Source: CAD feature listing. Evaluate the final solid. Frame: model axes, mm. A direction names the side the tool comes from. Coordinates: 2 decimals unless noted, no trailing zeros. Write each loop counter-clockwise with the first axis right and the second up, starting at its lowest first coordinate (ties: lowest second). Pieces come first, ordered by that corner, then holes. Notation, with made-up numbers: (-29.75, 12.5) - (-12.75, 12.5) arc R15 cw to (-12.75, 39.5) - close; hole circle Ø3 at (-10, 48). An arc over 180 degrees is marked (long way). One line per question, with ' | ' between items.
from build123d import *

# Parameters (mm, degrees)
SKETCH2_R               = 5
SKETCH2_R_2             = 3
BOSS_EXTRUDE1_DEPTH     = 20
CUT_EXTRUDE1_DEPTH      = 22.213203436
CUT_EXTRUDE1_DEPTH_BACK = 22.213203436
SKETCH3_R               = 1.25
BOSS_EXTRUDE2_DEPTH     = 8


with BuildPart() as part:
    # Sketch2 → Boss-Extrude1 (new body)
    with BuildSketch(Plane(origin=(0, 0, 0), x_dir=(1, 0, 0), z_dir=(0, 1, 0))):
        with Locations(Location((0, 0, 0), (0, 0, 270))):
            Circle(SKETCH2_R)
        with Locations(Location((0, 0, 0), (0, 0, 270))):
            Circle(SKETCH2_R_2, mode=Mode.SUBTRACT)
    extrude(amount=BOSS_EXTRUDE1_DEPTH)

    # Sketch3 → Cut-Extrude1 (cut, two sides: drawn at the far end of the back side and taken through both)
    with BuildSketch(Plane(origin=(0, 0, 0), x_dir=(0, 0, -1), z_dir=(1, 0, 0)).offset(-CUT_EXTRUDE1_DEPTH_BACK)):
        with Locations((0, 14)):
            Circle(SKETCH3_R)
    extrude(amount=CUT_EXTRUDE1_DEPTH + CUT_EXTRUDE1_DEPTH_BACK, mode=Mode.SUBTRACT)

    # Sketch4 → Boss-Extrude2 (add)
    with BuildSketch(Plane.XZ):
        with BuildLine():
            Line((11.223747146, -0.768114575), (14.074787242, 0.165464759))
            Line((14.074787242, 0.165464759), (11.202587609, 1.031761053))
            ThreePointArc((11.202587609, 1.031761053), (11.090038067, 1.890385058), (10.911778318, 2.737808237))
            Line((10.911778318, 2.737808237), (13.334786699, 4.506714787))
            Line((13.334786699, 4.506714787), (10.335462245, 4.443053024))
            ThreePointArc((10.335462245, 4.443053024), (9.963091861, 5.224873259), (9.531688601, 5.975735303))
            Line((9.531688601, 5.975735303), (11.289484326, 8.406816172))
            Line((11.289484326, 8.406816172), (8.456629826, 7.41942801))
            ThreePointArc((8.456629826, 7.41942801), (7.860888806, 8.047914461), (7.218570793, 8.628715763))
            Line((7.218570793, 8.628715763), (8.139088568, 11.483999816))
            Line((8.139088568, 11.483999816), (5.750003558, 9.669537687))
            ThreePointArc((5.750003558, 9.669537687), (4.989207185, 10.083169723), (4.19884898, 10.437057403))
            Line((4.19884898, 10.437057403), (4.191982112, 13.437049544))
            Line((4.191982112, 13.437049544), (2.48052688, 10.973125644))
            ThreePointArc((2.48052688, 10.973125644), (1.629147203, 11.131414079), (0.768114575, 11.223747146))
            Line((0.768114575, 11.223747146), (-0.165464759, 14.074787242))
            Line((-0.165464759, 14.074787242), (-1.031761053, 11.202587609))
            ThreePointArc((-1.031761053, 11.202587609), (-1.890385058, 11.090038067), (-2.737808237, 10.911778318))
            Line((-2.737808237, 10.911778318), (-4.506714787, 13.334786699))
            Line((-4.506714787, 13.334786699), (-4.443053024, 10.335462245))
            ThreePointArc((-4.443053024, 10.335462245), (-5.224873259, 9.963091861), (-5.975735303, 9.531688601))
            Line((-5.975735303, 9.531688601), (-8.406816172, 11.289484326))
            Line((-8.406816172, 11.289484326), (-7.41942801, 8.456629826))
            ThreePointArc((-7.41942801, 8.456629826), (-8.047914461, 7.860888806), (-8.628715763, 7.218570793))
            Line((-8.628715763, 7.218570793), (-11.483999816, 8.139088568))
            Line((-11.483999816, 8.139088568), (-9.669537687, 5.750003558))
            ThreePointArc((-9.669537687, 5.750003558), (-10.083169723, 4.989207185), (-10.437057403, 4.19884898))
            Line((-10.437057403, 4.19884898), (-13.437049544, 4.191982112))
            Line((-13.437049544, 4.191982112), (-10.973125644, 2.48052688))
            ThreePointArc((-10.973125644, 2.48052688), (-11.131414079, 1.629147203), (-11.223747146, 0.768114575))
            Line((-11.223747146, 0.768114575), (-14.074787242, -0.165464759))
            Line((-14.074787242, -0.165464759), (-11.202587609, -1.031761053))
            ThreePointArc((-11.202587609, -1.031761053), (-11.090038067, -1.890385058), (-10.911778318, -2.737808237))
            Line((-10.911778318, -2.737808237), (-13.334786699, -4.506714787))
            Line((-13.334786699, -4.506714787), (-10.335462245, -4.443053024))
            ThreePointArc((-10.335462245, -4.443053024), (-9.963091861, -5.224873259), (-9.531688601, -5.975735303))
            Line((-9.531688601, -5.975735303), (-11.289484326, -8.406816172))
            Line((-11.289484326, -8.406816172), (-8.456629826, -7.41942801))
            ThreePointArc((-8.456629826, -7.41942801), (-7.860888806, -8.047914461), (-7.218570793, -8.628715763))
            Line((-7.218570793, -8.628715763), (-8.139088568, -11.483999816))
            Line((-8.139088568, -11.483999816), (-5.750003558, -9.669537687))
            ThreePointArc((-5.750003558, -9.669537687), (-4.989207185, -10.083169723), (-4.19884898, -10.437057403))
            Line((-4.19884898, -10.437057403), (-4.191982112, -13.437049544))
            Line((-4.191982112, -13.437049544), (-2.48052688, -10.973125644))
            ThreePointArc((-2.48052688, -10.973125644), (-1.629147203, -11.131414079), (-0.768114575, -11.223747146))
            Line((-0.768114575, -11.223747146), (0.165464759, -14.074787242))
            Line((0.165464759, -14.074787242), (1.031761053, -11.202587609))
            ThreePointArc((1.031761053, -11.202587609), (1.890385058, -11.090038067), (2.737808237, -10.911778318))
            Line((2.737808237, -10.911778318), (4.506714787, -13.334786699))
            Line((4.506714787, -13.334786699), (4.443053024, -10.335462245))
            ThreePointArc((4.443053024, -10.335462245), (5.224873259, -9.963091861), (5.975735303, -9.531688601))
            Line((5.975735303, -9.531688601), (8.406816172, -11.289484326))
            Line((8.406816172, -11.289484326), (7.41942801, -8.456629826))
            ThreePointArc((7.41942801, -8.456629826), (8.047914461, -7.860888806), (8.628715763, -7.218570793))
            Line((8.628715763, -7.218570793), (11.483999816, -8.139088568))
            Line((11.483999816, -8.139088568), (9.669537687, -5.750003558))
            ThreePointArc((9.669537687, -5.750003558), (10.083169723, -4.989207185), (10.437057403, -4.19884898))
            Line((10.437057403, -4.19884898), (13.437049544, -4.191982112))
            Line((13.437049544, -4.191982112), (10.973125644, -2.48052688))
            ThreePointArc((10.973125644, -2.48052688), (11.131414079, -1.629147203), (11.223747146, -0.768114575))
        make_face()
    extrude(amount=-BOSS_EXTRUDE2_DEPTH)


solid = part.part
Item 1: Cut plane C-C on x = 9. Return loops of the section in (y, z).
Check sheet entries:
outline: (0, -7.34) - (8, -7.34) - (8, 7.61) - (0, 7.61) - close
Item 2: Pin query (flat end, axial travel): pin 1 Ø3 at (x, z) = (-0.5, 0) entering from +Y; pin 2 Ø1.5 at (y, z) = (13, 4) entering from -X; pin 3 Ø12 at (x, y) = (-5.5, 17.5) entering from -Z; pin 4 Ø1.5 at (y, z) = (17.5, -6) entering from +X. Return the tip coordinate at first contact, or that it passes through.
Check sheet entries:
pin 1: y = 8 | pin 2: x = -3.8 | pin 3: z = -5 | pin 4: through
Item 3: Mould query, pull axis Y, two halves, no side actions, for faces 1 (the face through (0, 0, 0)), 2 (the face through (3.85, 12.78, 0.27)), 3 (the face through (0.308, 3.944, 12.629)). Classes: pulls with the +Y half, pulls with the -Y half, needs draft (parallel to the pull), parting line crosses it, or undercut.
Check sheet entries:
face 1: pulls with the -Y half | face 2: undercut | face 3: needs draft
Item 4: Ray query, line 1 along Y through (x, z) = (-3.4, 0); line 2 along X through (y, z) = (15.5, 0). Return the intervals inside material, ascending. Write a range as [from, to].
Check sheet entries:
line 1: [0, 12.75], [15.25, 20] | line 2: [-5, -3], [3, 5]
Item 5: Cut plane A-A on y = 14.5. Return loops of the section in (x, z), and give its area (3 significant figures).
Check sheet entries:
outline: (-4.87, -1.15) arc R5 ccw to (4.87, -1.15) - (2.77, -1.15) arc R3 cw to (-2.77, -1.15) - close; (-4.87, 1.15) - (-2.77, 1.15) arc R3 cw to (2.77, 1.15) - (4.87, 1.15) arc R5 ccw to start | area: 41.0 mm²
Item 6: Access query for faces 4 (the face through (10.036, 3.944, -7.672)), 5 (the face through (-10.08, 3.94, 5)), 6 (the face through (3.348, 3.944, 12.222)), 7 (the face through (10.398, 3.944, 7.174)), 8 (the face through (-1.15, 13.92, 2.77)). Directions: +Z, -Z, +X, -X, +Y, -Y. A direction counts if a zero-diameter tool reaches every point of the face in a straight line with its end or side. Return the directions, or none.
Check sheet entries:
face 4: -Z, +Y, -Y | face 5: -X, +Y, -Y | face 6: +Z, +Y, -Y | face 7: +X, +Y, -Y | face 8: +Y
Item 7: Cut plane B-B on z = 9. Return loops of the section in (x, y).
Check sheet entries:
outline: (-7.61, 0) - (7.34, 0) - (7.34, 8) - (-7.61, 8) - close
